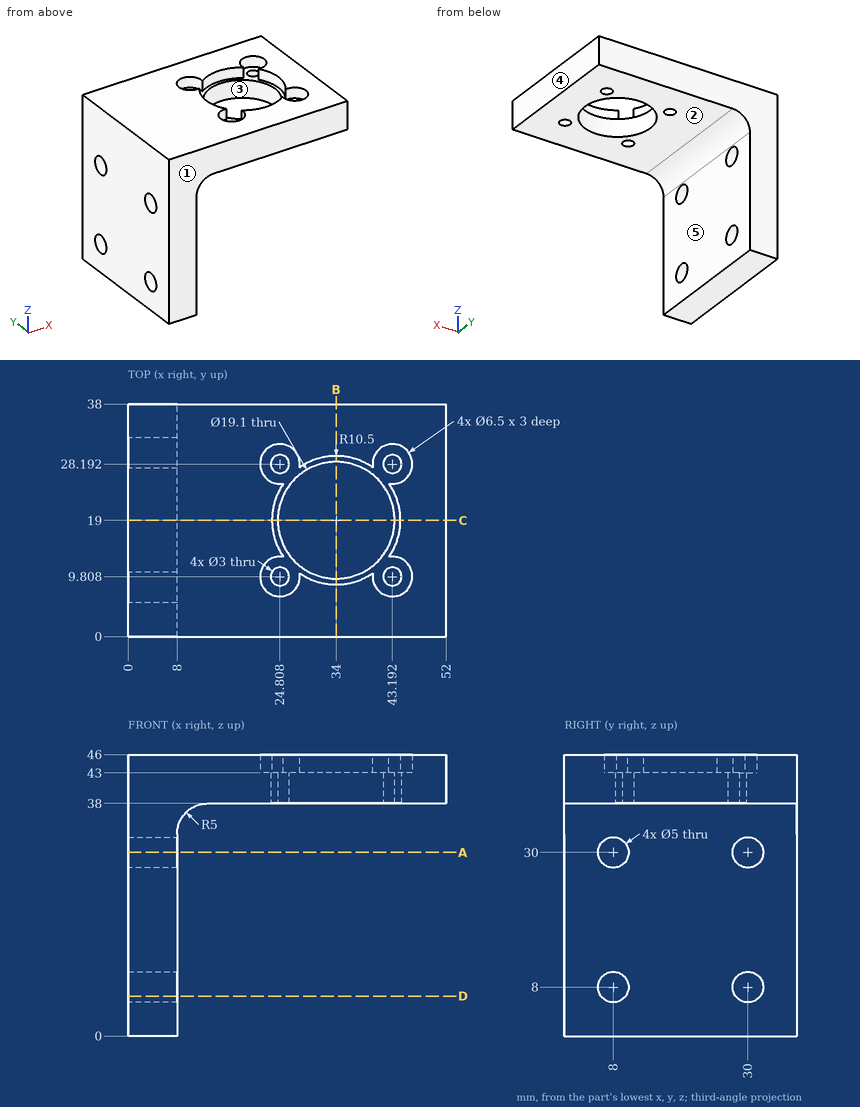
Check sheet for the drawn part. Datum: minimum x, y, z corner. Units: mm. A direction names the side the tool comes from. Give positions to 0.01 mm unless a question says otherwise; leave off trailing zeros. Order: outer loops, then holes, each group sorted by start corner. A loop starts at its lowest first (then second) coordinate and runs counter-clockwise, first axis right, second up. Notation, with made-up numbers: (2, 55.25) -> (36, 55.25) arc R29 cw to (36, 89.25) -> close; hole circle Ø10 at (72, 0). An arc over 180 degrees is marked (long way). One line per item, written item: value.
(1) Sectioned sample at B-B on x = 34. Record the cut outline in (y, z).
Final values:
outline: (0, 38) -> (9.45, 38) -> (9.45, 43) -> (8.5, 43) -> (8.5, 46) -> (0, 46) -> close; (28.55, 38) -> (38, 38) -> (38, 46) -> (29.5, 46) -> (29.5, 43) -> (28.55, 43) -> close
(2) Sectioned sample at C-C on y = 19. Record the cut outline in (x, z), then the cut area to 3 significant figures.
Final values:
outline: (0, 0) -> (8, 0) -> (8, 33) arc R5 cw to (13, 38) -> (24.45, 38) -> (24.45, 43) -> (23.5, 43) -> (23.5, 46) -> (0, 46) -> close; (43.55, 38) -> (52, 38) -> (52, 46) -> (44.5, 46) -> (44.5, 43) -> (43.55, 43) -> close
area: 567 mm^2
(3) Draft check along Y on the marked faces 1, 2 and 3. Enter one of: pulls with the +Y half, pulls with the -Y half, needs draft (parallel to the pull), parting line crosses it, or undercut.
Final values:
face 1: pulls with the -Y half
face 2: needs draft
face 3: undercut
(4) Tool access check on the marked faces 4 and 5. Record the directions out of +Z, -Z, +X, -X, +Y, -Y that give a thin tool (end or side, any length) a straight path to the whole face; none if there is none.
Final values:
face 4: +Z, -Z, +X, +Y, -Y
face 5: -Z, +X, +Y, -Y
(5) Scan lines: line 1 along Y through (x, z) = (3.5, 8); line 2 along X through (y, z) = (14, 31.5); line 3 along Z through (x, y) = (24.5, 35). Record each from-to range of solid material in increasing order. Write a range as [from, to].
Final values:
line 1: [0, 5.5], [10.5, 27.5], [32.5, 38]
line 2: [0, 8]
line 3: [38, 46]
(6) Gauge pin test, flat ends, axial feed: pin 1 (3 mm diameter, centred on y = 30, z = 30, fed in from +X); pin 2 (3.5 mm diameter, centred on x = 24.81, y = 9.81, fed in from -Z); pin 3 (1.5 mm diameter, centred on y = 34, z = 18, fed in from +X); pin 4 (5 mm diameter, centred on x = 24.81, y = 28.19, fed in from +Z). Record the tip position at first contact, or that the pin passes through.
Final values:
pin 1: through
pin 2: z = 38
pin 3: x = 8
pin 4: z = 43
(7) Sectioned sample at A-A on z = 30. Record the cut outline in (x, y).
Final values:
outline: (0, 0) -> (8, 0) -> (8, 5.5) -> (0, 5.5) -> close; (0, 10.5) -> (8, 10.5) -> (8, 27.5) -> (0, 27.5) -> close; (0, 32.5) -> (8, 32.5) -> (8, 38) -> (0, 38) -> close
(8) Sectioned sample at D-D on z = 6.5. Record the cut outline in (x, y), then the cut area to 3 significant figures.
Final values:
outline: (0, 0) -> (8, 0) -> (8, 6) -> (0, 6) -> close; (0, 10) -> (8, 10) -> (8, 28) -> (0, 28) -> close; (0, 32) -> (8, 32) -> (8, 38) -> (0, 38) -> close
area: 240 mm^2
